from build123d import *

# Parameters (mm, degrees)
CHANFREIN1_SIZE = 1


with BuildPart() as part:
    # Esquisse1 → Révolution1 (revolve)
    with BuildSketch(Plane.XY, mode=Mode.PRIVATE) as r_volution1_sk:
        Polygon((-25, 11), (25, 11), (25, 18), (5, 18), (5, 45), (19, 47), (19, 50), (-19, 50), (-19, 47), (-5, 45), (-5, 18), (-25, 18), align=None)
    revolve(r_volution1_sk.sketch.rotate(Axis((-40.635842881, 0, 0), (1, 0, 0)), 270), axis=Axis((-40.635842881, 0, 0), (1, 0, 0)))

    # Chanfrein1
    chanfrein1_edges = [part.edges().sort_by_distance(p)[0] for p in [
        (-25, 0, 11),
        (25, 0, 11),
    ]]
    chamfer(chanfrein1_edges, length=CHANFREIN1_SIZE)


solid = part.part
Read the model definition and answer for the solid it produces. Units are mm, in the model's axes. A direction names the side the tool comes from. Give positions to 0.01 mm unless a question says otherwise; leave off trailing zeros. Write each loop counter-clockwise with the first axis right and the second up, starting at its lowest first coordinate (ties: lowest second). Pieces come first, ordered by that corner, then holes. Notation, with made-up numbers: (19.5, 22) - (73.5, 22) arc R33 cw to (73.5, 58) - close; hole circle Ø3 at (51, 47.5). An arc over 180 degrees is marked (long way). Answer in a Markdown table with one row per item. Add a question column.
Item 1: Section A-A, the plane y = 0 is taken. Write down the section's boundary in (x, z).
Item 2: Determine the mould class of faces 1 (the face through (-19, -33, 34)), 2 (the face through (-5, -19, 1)), 3 (the face through (-0.27, 15.02, -47.69)) for opening direction Z: pulls with the +Z half, pulls with the -Z half, needs draft (parallel to the pull), parting line crosses it, or undercut.
Item 3: Section C-C, the plane x = 9 is taken. Write down the section's boundary in (y, z), and give its area (3 significant figures).
Item 4: A tool of negligible diameter and unlimited length cuts with its end or side. For faces 4 (the face through (0.34, -10.74, 2.38)), 5 (the face through (-15.14, 5.407, -17.169)), 6 (the face through (5, -19, -1)), from which of +Z, -Z, +X, -X, +Y, -Y can it reach the whole face along a straight path? Write none if from no direction.
Item 5: Section D-D, the plane x = 1 is taken. Write down the section's boundary in (y, z), and give its area (3 significant figures).
Item 6: Flat-ended cylindrical pins translate along their axes: P1, Ø6, axis at x = 11.5, y = 9, coming from the +Z side; P2, Ø5, axis at x = 16, z = 26, coming from the -Y side; P3, Ø5, axis at x = -1, z = -7.5, coming from the -Y side. Find the tip coordinate at first contact, or state that the pin passes through.
Item 7: Find the intervals of material crossed by L1, parallel to Y at x = 13.5, z = 0; L2, parallel to Y at x = -17, z = -3.5; L3, parallel to Z at x = -16, y = -9, in increasing order.
Recorded:
| question | item | result |
|---|---|---|
| 1 | outline | (-25, -18) - (-5, -18) - (-5, -45) - (-19, -47) - (-19, -50) - (19, -50) - (19, -47) - (5, -45) - (5, -18) - (25, -18) - (25, -12) - (24, -11) - (-24, -11) - (-25, -12) - close; (-25, 12) - (-24, 11) - (24, 11) - (25, 12) - (25, 18) - (5, 18) - (5, 45) - (19, 47) - (19, 50) - (-19, 50) - (-19, 47) - (-5, 45) - (-5, 18) - (-25, 18) - close |
| 2 | face 1 | needs draft |
| 2 | face 2 | undercut |
| 2 | face 3 | parting line crosses it |
| 3 | outline | circle Ø100 at (0, 0); circle Ø36 at (0, 0); hole circle Ø91.14 at (0, 0); hole circle Ø22 at (0, 0) |
| 3 | area | 1,970 mm2 |
| 4 | face 4 | +X, -X |
| 4 | face 5 | -X |
| 4 | face 6 | +X |
| 5 | outline | circle Ø100 at (0, 0); hole circle Ø22 at (0, 0) |
| 5 | area | 7,470 mm2 |
| 6 | P1 | stops at z = 49.64 |
| 6 | P2 | stops at y = -44.13 |
| 6 | P3 | stops at y = -49.75 |
| 7 | L1 | y = -50 to -46.21, -18 to -11, 11 to 18, 46.21 to 50 |
| 7 | L2 | y = -49.88 to -46.58, -17.66 to -10.43, 10.43 to 17.66, 46.58 to 49.88 |
| 7 | L3 | z = -49.18 to -45.69, -15.59 to -6.32, 6.32 to 15.59, 45.69 to 49.18 |
